Could you check a few things on this model? Use its own coordinates, in mm. A direction names the side the tool comes from. Round coordinates to 2 decimals unless told otherwise and drop trailing zeros. Loops run counter-clockwise (first coordinate to the right, second up) from the corner with the lowest first, then second, coordinate; pieces in that order, holes last. Notation, with made-up numbers: (-28.75, -17.5) - (5.25, -17.5) arc R20 cw to (5.25, -4.5) - close; hole circle Ø2 at (84, 61). An arc over 180 degrees is marked (long way). Answer as CSV lines item,"result". Start each with the question number.
1) Which directions (+Z, -Z, +X, -X, +Y, -Y) give clear straight access to the entire face, cutting with the end or side of a thin tool? Please do faces 5 (the face through (0, 252, 9.525)), 6 (the face through (0, 241, -12.7)).
2) We'd pull the mould along X, two halves only. Please class faces 1 (the face through (12.7, 254, 0)), 2 (the face through (0, 254, 12.7)), 3 (the face through (-12.7, 254, 0)), 4 (the face through (9.525, 252, 0)): pulls with the +X half, pulls with the -X half, needs draft (parallel to the pull), parting line crosses it, or undercut.
3) Please list where these lines run through material, in increasing order: line 1 along Y through (x, z) = (-10.5, 0); line 2 along Z through (x, y) = (-11.6, 63.5); line 3 along X through (y, z) = (90.5, -1.5) (3 decimals).
4) I'm going to push a flat-ended pin straight in: pin 1 Ø10 at (x, z) = (-6.5, -10) entering from +Y. Where does the tip first touch, or does it pass through?
5) Suppose I cut it at A-A, the plane y = 445.5. Write out the boundary of the cut face in (x, z) (3 decimals).
Autodesk Inventor part; units mm, degrees
ref_plane "YZ Plane" through (0, 0, 0) normal (1, 0, 0) x (0, 1, 0)
ref_plane "XZ Plane" through (0, 0, 0) normal (0, 1, 0) x (-1, 0, 0)
ref_plane "XY Plane" through (0, 0, 0) normal (0, 0, 1) x (1, 0, 0)
sketch "Sketch1" plane through (0, 0, 0) normal (0, 1, 0) x (-1, 0, 0)
  line L0 (-12.7, -12.7) -> (12.7, -12.7)
  line L1 (12.7, -12.7) -> (12.7, 12.7)
  line L2 (12.7, 12.7) -> (-12.7, 12.7)
  line L3 (-12.7, 12.7) -> (-12.7, -12.7)
  line L4 (-12.7, -12.7) -> (12.7, 12.7) construction
  line L5 (12.7, -12.7) -> (-12.7, 12.7) construction
  line L6 (9.525, 9.525) -> (9.525, -9.525)
  line L7 (9.525, -9.525) -> (-9.525, -9.525)
  line L8 (-9.525, -9.525) -> (-9.525, 9.525)
  line L9 (-9.525, 9.525) -> (9.525, 9.525)
  point P0 (0, 0)
  dimension "d0" = 25.4
  dimension "d1" = 25.4
  dimension "d2" = 3.175
extrude "Extrusion1" add sketch "Sketch1" along normal blind 514.35
sketch "Sketch2" plane through (12.7, 0, 12.7) normal (1, 0, 0) x (0, 0, -1)
  line L0 (25.4, 514.35) -> (0, 514.35)
  line L1 (0, 514.35) -> (25.4, 488.95)
  line L2 (25.4, 0) -> (25.4, 514.35)
  circle A0 centre (12.7, 482.6) radius 3.2512
  line L3 (0, 514.35) -> (25.4, 514.35)
  circle A1 centre (12.7, 463.55) radius 3.2512
  circle A2 centre (12.7, 501.65) radius 3.2512
  point P0 (12.7, 0)
  point P1 (12.7, 514.35)
  point P2 (12.7, 514.35)
  point P3 (14.9989, 499.3511)
  point P4 (10.4011, 503.9489)
  dimension "d5" = 25.4
  dimension "d6" = 6.5024
  dimension "d7" = 31.75
  dimension "d8" = 19.05
extrude "Extrusion2" cut sketch "Sketch2" against normal blind 522.224
sketch "Sketch5" plane through (12.7, 0, -12.7) normal (0, 0, -1) x (-1, 0, 0)
  circle A0 centre (12.7, 209.55) radius 3.2512
  line L0 (0, 0) -> (25.4, 0)
  line L1 (25.4, 514.35) -> (0, 514.35)
  point P0 (12.7, 0)
  point P1 (12.7, 0)
  point P2 (12.7, 514.35)
  dimension "d11" = 6.5024
  dimension "d15" = 304.8
extrude "Extrusion3" cut sketch "Sketch5" against normal blind 25.4
sketch "Sketch6" plane through (-12.7, 0, -12.7) normal (-1, 0, 0) x (0, 0, 1)
  line L0 (12.7, 0) -> (12.7, 63.5)
  circle A0 centre (12.7, 63.5) radius 2.4892
  dimension "d16" = 63.5
  dimension "d17" = 4.9784
extrude "Extrusion4" cut sketch "Sketch6" against normal blind 25.4
properties part number "STRU_002_BilletPole_20.56in_Angled" material "Aluminum 6061"
Filled sheet:
1,face 5,"+Y, -Y"
1,face 6,"-Z, +X, -X, +Y, -Y"
2,face 1,"pulls with the +X half"
2,face 2,"needs draft"
2,face 3,"pulls with the -X half"
2,face 4,"undercut"
3,line 1,"0 to 61.01, 65.99 to 460.3, 466.8 to 479.35, 485.85 to 498.4"
3,line 2,"-12.7 to -2.49, 2.49 to 12.7"
3,line 3,"-12.7 to -9.525, 9.525 to 12.7"
4,pin 1,"y = 495.63"
5,outline,"(-12.7, -12.7) - (12.7, -12.7) - (12.7, 12.7) - (-12.7, 12.7) - close; hole (-9.525, -9.525) - (9.525, -9.525) - (9.525, 9.525) - (-9.525, 9.525) - close"
